```python
from build123d import *

# Parameters (mm, degrees)
SKETCH1_R           = 1.9
SKETCH1_R_2         = 4.2
BOSS_EXTRUDE1_DEPTH = 10
SKETCH2_R           = 12
BOSS_EXTRUDE2_DEPTH = 7
SKETCH3_R           = 11.2
CUT_EXTRUDE1_DEPTH  = 7
SKETCH4_R           = 2.9
CUT_EXTRUDE2_DEPTH  = 2


with BuildPart() as part:
    # Sketch1 → Boss-Extrude1 (new body)
    with BuildSketch(Plane(origin=(0, 0, 0), x_dir=(0, 1, 0), z_dir=(0, 0, 1))):
        with BuildLine():
            Line((0, 19.038851754), (70, 19.038851754))
            Line((70, 19.038851754), (70, -19.038851754))
            Line((70, -19.038851754), (69.469297143, -19.038851754))
            Line((69.469297143, -19.038851754), (68.091336606, -23.038851754))
            ThreePointArc((68.091336606, -23.038851754), (64.091336606, -25.891585633), (60.091336606, -23.038851754))
            Line((60.091336606, -23.038851754), (56.091336606, -19.038851754))
            Line((56.091336606, -19.038851754), (0, -19.038851754))
            ThreePointArc((0, -19.038851754), (-19.038851754, 0), (0, 19.038851754))
        make_face()
        with Locations(Location((0, 14.242669761, 0), (0, 0, 270))):
            Circle(SKETCH1_R, mode=Mode.SUBTRACT)
        with Locations(Location((0, 0, 0), (0, 0, 270))):
            Circle(SKETCH1_R_2, mode=Mode.SUBTRACT)
        with Locations(Location((0, -14.242669761, 0), (0, 0, 90))):
            Circle(SKETCH1_R, mode=Mode.SUBTRACT)
        with Locations(Location((-14.537854627, 0, 0), (0, 0, 270))):
            Circle(SKETCH1_R, mode=Mode.SUBTRACT)
        with Locations(Location((14.537854627, 0, 0), (0, 0, 90))):
            Circle(SKETCH1_R, mode=Mode.SUBTRACT)
        with Locations(Location((64.091336606, -21.660891217, 0), (0, 0, 270))):
            Circle(SKETCH1_R, mode=Mode.SUBTRACT)
        with Locations(Location((42.352384866, 12.099919194, 0), (0, 0, 270))):
            Circle(SKETCH1_R, mode=Mode.SUBTRACT)
        with Locations(Location((55.398759947, 5.77203667, 0), (0, 0, 270))):
            Circle(SKETCH1_R, mode=Mode.SUBTRACT)
    extrude(amount=BOSS_EXTRUDE1_DEPTH)

    # Sketch2 → Boss-Extrude2 (add)
    with BuildSketch(Plane(origin=(0, 0, 0), x_dir=(1, 0, 0), z_dir=(0, 0, -1))):
        Circle(SKETCH2_R)
    extrude(amount=BOSS_EXTRUDE2_DEPTH)

    # Sketch3 → Cut-Extrude1 (cut)
    with BuildSketch(Plane(origin=(0, 0, -7), x_dir=(1, 0, 0), z_dir=(0, 0, -1))):
        with Locations(Location((0, 0, 0), (0, 0, 180))):
            Circle(SKETCH3_R)
    extrude(amount=-CUT_EXTRUDE1_DEPTH, mode=Mode.SUBTRACT)

    # Sketch4 → Cut-Extrude2 (cut)
    with BuildSketch(Plane(origin=(0, 0, 0), x_dir=(1, 0, 0), z_dir=(0, 0, -1))):
        with Locations(Location((-12.099919194, -42.352384866, 0), (0, 0, 180))):
            Circle(SKETCH4_R)
        with Locations(Location((-5.77203667, -55.398759947, 0), (0, 0, 180))):
            Circle(SKETCH4_R)
    extrude(amount=-CUT_EXTRUDE2_DEPTH, mode=Mode.SUBTRACT)


solid = part.part
```
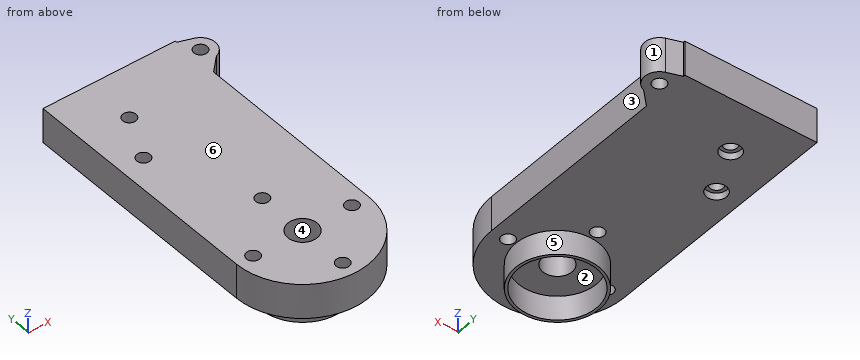
Geometry check sheet. Reference: the model listing, model coordinates, mm. Face numbers are marked on the shaded views. A direction names the side the tool comes from. Give positions to 0.01 mm unless a question says otherwise; leave off trailing zeros. Order: outer loops, then holes, each group sorted by start corner. A loop starts at its lowest first (then second) coordinate and runs counter-clockwise, first axis right, second up.
1. Thickness scan on L1, parallel to Y at x = 0, z = 4.75; L2, parallel to Y at x = -1.5, z = 5.25; L3, parallel to X at y = 25, z = 5.5. Record the ranges inside material, lowest first.
2. Gauge pin test, flat ends, axial feed: pin 1 Ø4.5 at (x, y) = (-6, 54.5) entering from -Z; pin 2 Ø6 at (x, z) = (0.5, 6) entering from -Y; pin 3 Ø3 at (y, z) = (35, 7) entering from +X. Record the tip position at first contact, or that the pin passes through.
3. Access from +Z, -Z, +X, -X, +Y, -Y to the whole of each face (thin tool, end or side, straight path). Record for the marked faces 1, 2 and 3.
4. Section check A-A, the plane x = 0. Enter the section's corners in (y, z).
5. Section check C-C, the plane y = 34. Enter the section's corners in (x, z).
6. Release check for a two-part mould opening along Y. For the marked faces 4, 5 and 6 record: pulls with the +Y half, pulls with the -Y half, needs draft (parallel to the pull), parting line crosses it, or undercut.
7. Section check B-B, the plane z = -1.25. Enter the section's corners in (x, y).
Values follow:
1. L1: y = -19.04 to -16.44, -12.64 to -4.2, 4.2 to 12.64, 16.44 to 70
1. L2: y = -18.98 to -15.7, -13.37 to -3.92, 3.92 to 13.37, 15.7 to 70
1. L3: x = -19.04 to 19.04
2. pin 1: stops at z = 0
2. pin 2: stops at y = -19.04
2. pin 3: stops at x = 19.04
3. face 1: +Z, -Z, +X
3. face 2: -Z
3. face 3: +Z, -Z, +X, -Y
4. outline: (-19.04, 0) - (-16.44, 0) - (-16.44, 10) - (-19.04, 10) - close; (-12.64, 0) - (-12, 0) - (-12, -7) - (-11.2, -7) - (-11.2, 0) - (-4.2, 0) - (-4.2, 10) - (-12.64, 10) - close; (4.2, 0) - (11.2, 0) - (11.2, -7) - (12, -7) - (12, 0) - (12.64, 0) - (12.64, 10) - (4.2, 10) - close; (16.44, 0) - (70, 0) - (70, 10) - (16.44, 10) - close
5. outline: (-19.04, 0) - (19.04, 0) - (19.04, 10) - (-19.04, 10) - close
6. face 4: undercut
6. face 5: parting line crosses it
6. face 6: needs draft
7. outline: circle Ø24 at (0, 0); hole circle Ø22.4 at (0, 0)
